```python
from build123d import *

# Parameters (mm, degrees)
F1_DEPTH = 88.646
F2_R     = 12.877415
F3_R     = 26.981251
F4_SIZE  = 5.08


with BuildPart() as f1:
    # F0 (on Front) → F1 (new body)
    with BuildSketch(Plane.XZ):
        Polygon((-35.384025, 45.681097), (-68.046205, 45.681097), (-68.046205, 0), (-8.452052, 0), (-8.452052, 25.599297), (24.783138, 25.599297), (24.783138, 72.478622), (-35.384025, 72.478622), align=None)
    extrude(amount=F1_DEPTH)

    # F2
    f2_edges = [f1.edges().sort_by_distance(p)[0] for p in [
        (24.783138, -44.323, 72.478622),
        (-35.384025, -44.323, 72.478622),
    ]]
    fillet(f2_edges, radius=F2_R)

    # F3
    f3_edges = [f1.edges().sort_by_distance(p)[0] for p in [
        (-35.384025, -44.323, 45.681097),
    ]]
    fillet(f3_edges, radius=F3_R)

    # F4
    f4_edges = [f1.edges().sort_by_distance(p)[0] for p in [
        (-68.046205, -44.323, 45.681097),
    ]]
    chamfer(f4_edges, length=F4_SIZE)


solid = f1.part
```
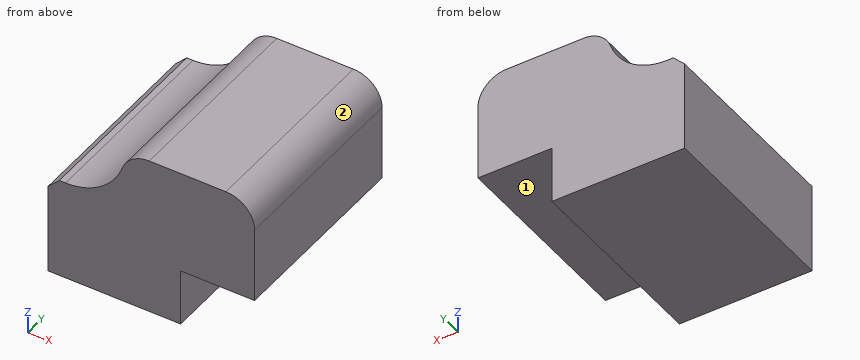
CAD build for the part. Positions are in the model's coordinates, mm. Face numbers are marked on the shaded views. A direction names the side the tool comes from. Give positions to 0.01 mm unless a question says otherwise; leave off trailing zeros. Order: outer loops, then holes, each group sorted by start corner. A loop starts at its lowest first (then second) coordinate and runs counter-clockwise, first axis right, second up. Notation, with made-up numbers: M 57,42.25 L 72,42.25 A24 cw 72,52.25 Z; hole C 35.5,9 d1. An arc over 180 degrees is marked long. Put each result on its own line as item: value. Start each with the question number.
(1) Drill centre lines: line 1 along X through (y, z) = (-73.5, 21); line 2 along Z through (x, y) = (11, -36.5); line 3 along Z through (x, y) = (-56.5, -68). Where is each one in solid material? Low to high.
(2) Flat gauge pins, fed straight in: pin 1 Ø2 at (x, y) = (-62, -62) entering from +Z; pin 2 Ø5 at (y, z) = (-77.5, 8) entering from +X; pin 3 Ø1 at (y, z) = (-14, 50.5) entering from -X. Where does each tip first touch, or does it go through?
(3) Saw through at B-B, the plane z = 42. Write the cut outline in (x, y).
(4) Saw through at A-A, the plane x = 8. Write the cut outline in (y, z).
(5) Which spindle directions (+Z, -Z, +X, -X, +Y, -Y) get a long thin tool onto all of the face, cutting with end or side? Do the marked faces 1 and 2. Say none if no direction does.
Check result:
1. line 1: x = -68.05 to -8.45
1. line 2: z = 25.6 to 72.48
1. line 3: z = 0 to 45.93
2. pin 1: stops at z = 45.68
2. pin 2: stops at x = -8.45
2. pin 3: stops at x = -45.52
3. outline: M -66.65,-88.65 L 24.78,-88.65 L 24.78,0 L -66.65,0 Z
4. outline: M -88.65,25.6 L 0,25.6 L 0,72.48 L -88.65,72.48 Z
5. face 1: -Z, +X, +Y, -Y
5. face 2: +Z, +X, +Y, -Y
